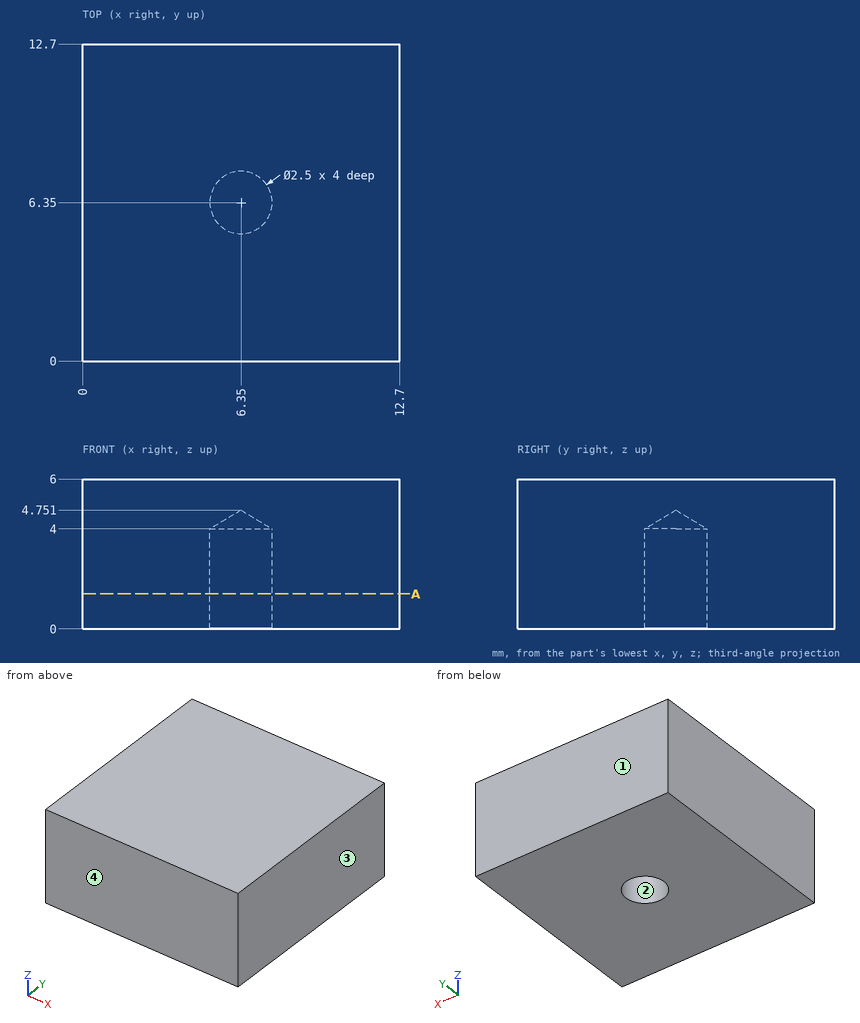
Geometry check sheet. Reference: drawing and pictorial views, mm from the part's lowest x, y, z. Give positions to 0.01 mm unless a question says otherwise; leave off trailing zeros. Order: outer loops, then holes, each group sorted by start corner. A loop starts at its lowest first (then second) coordinate and runs counter-clockwise, first axis right, second up. Notation, with made-up numbers: M -6.75,59 L 15.25,59 A20 ccw 15.25,89 Z; hole C 73.25,41.25 d1. An arc over 180 degrees is marked long. Return JSON: item names as keys, results as strings. Group by question number.
1) Scan lines: line 1 (X direction, y = 6.35, z = 2.25); line 2 (Y direction, x = 7.25, z = 0.55). Record each from-to range of solid material in increasing order.
2) Section check A-A on z = 1.4. Record the cut outline in (x, y), and give its area (3 significant figures).
3) Mould release check, pull along Y, two halves, no side actions. Record for the marked faces 1, 2, 3 and 4: pulls with the +Y half, pulls with the -Y half, needs draft (parallel to the pull), parting line crosses it, or undercut.
Answer block:
{
 "1": {"line 1": "x = 0 to 5.1, 7.6 to 12.7", "line 2": "y = 0 to 5.48, 7.22 to 12.7"},
 "2": {"outline": "M 0,0 L 12.7,0 L 12.7,12.7 L 0,12.7 Z; hole C 6.35,6.35 d2.5", "area": "156 mm^2"},
 "3": {"face 1": "pulls with the +Y half", "face 2": "undercut", "face 3": "needs draft", "face 4": "pulls with the -Y half"}
}
